Model file for the job. Use its own axes, mm. Face numbers are marked on the shaded views. A direction names the side the tool comes from. Round coordinates to 2 decimals unless told otherwise and drop trailing zeros. Order: outer loops, then holes, each group sorted by start corner. A loop starts at its lowest first (then second) coordinate and runs counter-clockwise, first axis right, second up. Notation, with made-up numbers: (66.25, -6) - (109.25, -6) arc R22 ccw to (109.25, 15) - close; hole circle Ø7 at (19.5, 54.5). An arc over 180 degrees is marked (long way). Put each result on its own line as item: value. Start each with the question number.
Item 1: Saw through at B-B on x = -18. List the corners of the cut face in (y, z).
Item 2: Which spindle directions (+Z, -Z, +X, -X, +Y, -Y) get a long thin tool onto all of the face, cutting with end or side? Do the marked faces 1, 2 and 3. Say none if no direction does.
Item 3: Mould opens along Y. For the marked faces 4, 5 and 6 say: pulls with the +Y half, pulls with the -Y half, needs draft (parallel to the pull), parting line crosses it, or undercut.
Item 4: Pin check, flat tips, straight feed: pin 1 Ø5.5 at (x, z) = (-23.5, 22) entering from -Y; pin 2 Ø0.6 at (y, z) = (6.5, 16.5) entering from +X; pin 3 Ø1.5 at (y, z) = (1.5, 16.5) entering from +X; pin 4 Ø1.4 at (y, z) = (7, 7) entering from +X. Stop position of each tip, or through.
Item 5: Saw through at A-A on y = 0. State how many separate pieces and enclosed holes the cut face has, plus the area to 3 significant figures.
Item 6: Saw through at C-C on z = 21.5. List the corners of the cut face in (x, y), plus the area to 3 significant figures.
Item 7: Saw through at D-D on x = -30. List the corners of the cut face in (y, z), plus the area to 3 significant figures.
Item 8: Probe probe 1 along Y at (x, z) = (0, 0.9); probe 2 along Y at (x, z) = (-23, 19); probe 3 along Z at (x, y) = (-30, 3.5). List the from-to ranges inside material, lowest first.
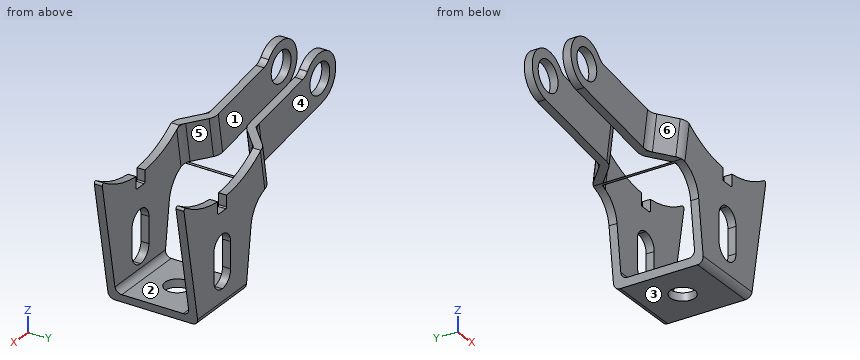
```python
from build123d import *

# Parameters (mm, degrees)
F1_DEPTH       = 7.3
F1_DEPTH_BACK  = 7.3
F3_DEPTH       = 6
F3_DEPTH_BACK  = 6
F5_DEPTH       = 10
F5_DEPTH_BACK  = 10
F8_DEPTH       = 25
F9_R           = 2.5
F10_DEPTH      = 10
F10_DEPTH_BACK = 10
F11_T1_DEPTH   = 6.5
F11_T6_DEPTH   = 12.7132034356
F11_S7_R       = 5
F11_T8_DEPTH   = 8
F11_S10_R      = 17
F11_T11_DEPTH  = 8
F11_T15_DEPTH  = 8.5710678119
F11_T20_DEPTH  = 12.7132034356
F11_S21_R      = 5
F11_T22_DEPTH  = 8
F11_S24_R      = 17
F11_T25_DEPTH  = 8
F11_T29_DEPTH  = 8.5710678119
F11_T31_DEPTH  = 10.6421356237
F12_R          = 1
F13_R          = 2
F14_DEPTH      = 5


# Not quite as in the source:
# - a fillet or chamfer that OpenCascade refuses, or shapes differently, is made with other operations: its cross-section is extruded or revolved along the edge and cut away or added


with BuildPart() as f1:
    # F0 (on Front) → F1 (new body, two sides)
    with BuildSketch(Plane.XZ) as f1_sk:
        with BuildLine():
            Line((-7.2480415045, 9.479816391), (-6, 0))
            Line((-6, 0), (6, 0))
            Line((6, 0), (9.6197658273, 19.3731186918))
            ThreePointArc((9.6197658273, 19.3731186918), (9.492555749, 19.6769779623), (9.1631662961, 19.6809084286))
            ThreePointArc((9.1631662961, 19.6809084286), (-0.3536100614, 17.0036780472), (-9.750799418, 20.0744152471))
            Line((-9.750799418, 20.0744152471), (-25.666835692, 22.7954629152))
            ThreePointArc((-25.666835692, 22.7954629152), (-26.3420622378, 23.0419468668), (-26.8865335991, 23.511240126))
            ThreePointArc((-26.8865335991, 23.511240126), (-33.4498266444, 23.0245236782), (-30.6740705867, 17.0572054525))
            Line((-30.6740705867, 17.0572054525), (-11.362677578, 13.7556786143))
            ThreePointArc((-11.362677578, 13.7556786143), (-8.6024605414, 12.2941429125), (-7.2480415045, 9.479816391))
        make_face()
    extrude(amount=F1_DEPTH)
    extrude(f1_sk.sketch, amount=-F1_DEPTH_BACK)

    # F2 (on Front) → F3 (cut, two sides)
    with BuildSketch(Plane.XZ) as f3_sk:
        Polygon((15, 1.3), (15, 78.0352148958), (0, 78.0352148958), (-11, 13.6936742961), (-11, 1.3), align=None)
    extrude(amount=F3_DEPTH, mode=Mode.SUBTRACT)
    extrude(f3_sk.sketch, amount=-F3_DEPTH_BACK, mode=Mode.SUBTRACT)

    # F4 (on Front) → F5 (cut, two sides)
    with BuildSketch(Plane.XZ) as f5_sk:
        with BuildLine():
            Line((0, 18), (-1.125, 18))
            Line((-1.125, 18), (-1.125, 15.2))
            ThreePointArc((-1.125, 15.2), (-1.0664213562, 15.0585786438), (-0.925, 15))
            Line((-0.925, 15), (0, 15))
            Line((0, 15), (0.925, 15))
            ThreePointArc((0.925, 15), (1.0664213562, 15.0585786438), (1.125, 15.2))
            Line((1.125, 15.2), (1.125, 18))
            Line((1.125, 18), (0, 18))
        make_face()
        with BuildLine():
            ThreePointArc((0, 11.5), (-1.50260191, 10.87760191), (-2.125, 9.375))
            Line((-2.125, 9.375), (-2.125, 5.125))
            ThreePointArc((-2.125, 5.125), (-1.50260191, 3.62239809), (0, 3))
            ThreePointArc((0, 3), (1.50260191, 3.62239809), (2.125, 5.125))
            Line((2.125, 5.125), (2.125, 9.375))
            ThreePointArc((2.125, 9.375), (1.50260191, 10.87760191), (0, 11.5))
        make_face()
    extrude(amount=F5_DEPTH, mode=Mode.SUBTRACT)
    extrude(f5_sk.sketch, amount=-F5_DEPTH_BACK, mode=Mode.SUBTRACT)

    # F7 (on offset) → F8 (cut)
    with BuildSketch(Plane(origin=(1.9622434031, 0, 11.4776148716), x_dir=(0.9856986369, 0, -0.1685176467), z_dir=(-0.1685176467, 0, -0.9856986369))):
        Polygon((-41.9907133171, -7.3), (-13.6887884036, -7.3), (-17.1887884036, -3.8), (-41.9907133171, -3.8), align=None)
        Polygon((-41.9907133171, 7.3), (-41.9907133171, 3.8), (-17.1887884036, 3.8), (-13.6887884036, 7.3), align=None)
        Polygon((-16.6503107725, -2.5), (-13.1503107725, -6), (-13.1503107725, 0), (-13.1503107725, 6), (-16.6503107725, 2.5), (-41.9907133171, 2.5), (-41.9907133171, 0), (-41.9907133171, -2.5), align=None)
    extrude(amount=-F8_DEPTH, mode=Mode.SUBTRACT)

    # F9 (on Front) → F10 (cut, two sides)
    with BuildSketch(Plane.XZ) as f10_sk:
        with Locations((-30, 21)):
            Circle(F9_R)
    extrude(amount=F10_DEPTH, mode=Mode.SUBTRACT)
    extrude(f10_sk.sketch, amount=-F10_DEPTH_BACK, mode=Mode.SUBTRACT)

    # F11: fillet of radius 2 on 8 edges, made by hand

    # F11_s2 → F11_t1 (join)
    with BuildSketch(Plane(origin=(1.9622434031, 0, 11.4776148716), x_dir=(0, 1, 0), z_dir=(0.1685176467, 0, 0.9856986369))):
        with BuildLine():
            ThreePointArc((3.8, 18.0172155284), (3.952240935, 17.2518486636), (4.3857864376, 16.603001966))
            Line((4.3857864376, 16.603001966), (3.8, 17.1887884036))
            Line((3.8, 17.1887884036), (3.8, 18.0172155284))
        make_face()
        with BuildLine():
            ThreePointArc((-4.3857864376, 16.603001966), (-3.952240935, 17.2518486636), (-3.8, 18.0172155284))
            Line((-3.8, 18.0172155284), (-3.8, 17.1887884036))
            Line((-3.8, 17.1887884036), (-4.3857864376, 16.603001966))
        make_face()
    extrude(amount=F11_T1_DEPTH)


with BuildPart() as f11_tool4:
    # F11_s5 → F11_t6 (new body)
    with BuildSketch(Plane(origin=(3.0576081065, 0, 17.8846560114), x_dir=(0, 1, 0), z_dir=(-0.1685176467, 0, -0.9856986369))):
        with BuildLine():
            ThreePointArc((-6, -12.3218836478), (-5.847759065, -13.0872505125), (-5.4142135624, -13.7360972102))
            Line((-5.4142135624, -13.7360972102), (-6, -13.1503107725))
            Line((-6, -13.1503107725), (-6, -12.3218836478))
        make_face()
    extrude(amount=F11_T6_DEPTH)

    # F11_s7 → F11_t8 (cut, symmetric)
    with BuildSketch(Plane.XZ.offset(5.7)):
        with Locations((-12.2052658114, 8.8271854299)):
            Circle(F11_S7_R)
    extrude(amount=F11_T8_DEPTH, both=True, mode=Mode.SUBTRACT)

    split(bisect_by=Plane.YZ.offset(-11), keep=Keep.TOP)

    # F11_s10 → F11_t11 (cut, symmetric)
    with BuildSketch(Plane.XZ.offset(5.7)):
        with Locations((0, 34)):
            Circle(F11_S10_R)
    extrude(amount=F11_T11_DEPTH, both=True, mode=Mode.SUBTRACT)


with BuildPart() as f1_1:
    add(f1.part)

    # F11_t3: union F11_tool4
    add(f11_tool4.part)


with BuildPart() as f11_tool13:
    # F11_s14 → F11_t15 (new body)
    with BuildSketch(Plane(origin=(3.4066195803, 0, 19.9261047304), x_dir=(0, 1, 0), z_dir=(-0.1685176467, 0, -0.9856986369))):
        with BuildLine():
            ThreePointArc((-6, -12.3218836478), (-5.847759065, -13.0872505125), (-5.4142135624, -13.7360972102))
            Line((-5.4142135624, -13.7360972102), (-6, -13.1503107725))
            Line((-6, -13.1503107725), (-6, -12.3218836478))
        make_face()
    extrude(amount=F11_T15_DEPTH)

    split(bisect_by=Plane.YZ.offset(-11), keep=Keep.BOTTOM)


with BuildPart() as f1_2:
    add(f1_1.part)

    # F11_t12: union F11_tool13
    add(f11_tool13.part)


with BuildPart() as f11_tool18:
    # F11_s19 → F11_t20 (new body)
    with BuildSketch(Plane(origin=(3.0576081065, 0, 17.8846560114), x_dir=(0, 1, 0), z_dir=(-0.1685176467, 0, -0.9856986369))):
        with BuildLine():
            ThreePointArc((6, -12.3218836478), (5.847759065, -13.0872505125), (5.4142135624, -13.7360972102))
            Line((5.4142135624, -13.7360972102), (6, -13.1503107725))
            Line((6, -13.1503107725), (6, -12.3218836478))
        make_face()
    extrude(amount=F11_T20_DEPTH)

    # F11_s21 → F11_t22 (cut, symmetric)
    with BuildSketch(Plane.XZ.offset(-5.7)):
        with Locations((-12.2052658114, 8.8271854299)):
            Circle(F11_S21_R)
    extrude(amount=F11_T22_DEPTH, both=True, mode=Mode.SUBTRACT)

    split(bisect_by=Plane.YZ.offset(-11), keep=Keep.TOP)

    # F11_s24 → F11_t25 (cut, symmetric)
    with BuildSketch(Plane.XZ.offset(-5.7)):
        with Locations((0, 34)):
            Circle(F11_S24_R)
    extrude(amount=F11_T25_DEPTH, both=True, mode=Mode.SUBTRACT)


with BuildPart() as f1_3:
    add(f1_2.part)

    # F11_t17: union F11_tool18
    add(f11_tool18.part)


with BuildPart() as f11_tool27:
    # F11_s28 → F11_t29 (new body)
    with BuildSketch(Plane(origin=(3.4066195803, 0, 19.9261047304), x_dir=(0, 1, 0), z_dir=(-0.1685176467, 0, -0.9856986369))):
        with BuildLine():
            ThreePointArc((6, -12.3218836478), (5.847759065, -13.0872505125), (5.4142135624, -13.7360972102))
            Line((5.4142135624, -13.7360972102), (6, -13.1503107725))
            Line((6, -13.1503107725), (6, -12.3218836478))
        make_face()
    extrude(amount=F11_T29_DEPTH)

    split(bisect_by=Plane.YZ.offset(-11), keep=Keep.BOTTOM)


with BuildPart() as f1_4:
    add(f1_3.part)

    # F11_t26: union F11_tool27
    add(f11_tool27.part)

    # F11_s32 → F11_t31 (cut)
    with BuildSketch(Plane(origin=(1.6132319293, 0, 9.4361661525), x_dir=(0, 1, 0), z_dir=(0.1685176467, 0, 0.9856986369))):
        with BuildLine():
            ThreePointArc((6.7142135624, 14.2745748413), (7.147759065, 13.6257281436), (7.3, 12.8603612789))
            Line((7.3, 12.8603612789), (7.3, 13.6887884036))
            Line((7.3, 13.6887884036), (6.7142135624, 14.2745748413))
        make_face()
        with BuildLine():
            ThreePointArc((-2.5, 17.4787378973), (-2.652240935, 16.7133710326), (-3.0857864376, 16.0645243349))
            Line((-3.0857864376, 16.0645243349), (-2.5, 16.6503107725))
            Line((-2.5, 16.6503107725), (-2.5, 17.4787378973))
        make_face()
        with BuildLine():
            ThreePointArc((-6.7142135624, 14.2745748413), (-7.147759065, 13.6257281436), (-7.3, 12.8603612789))
            Line((-7.3, 12.8603612789), (-7.3, 13.6887884036))
            Line((-7.3, 13.6887884036), (-6.7142135624, 14.2745748413))
        make_face()
        with BuildLine():
            ThreePointArc((2.5, 17.4787378973), (2.652240935, 16.7133710326), (3.0857864376, 16.0645243349))
            Line((3.0857864376, 16.0645243349), (2.5, 16.6503107725))
            Line((2.5, 16.6503107725), (2.5, 17.4787378973))
        make_face()
    extrude(amount=F11_T31_DEPTH, mode=Mode.SUBTRACT)

    # F12
    f12_edges = [f1_4.edges().sort_by_distance(p)[0] for p in [
        (0.035875, 6, 1.3),
        (0, -7.3, 0),
        (0.035875, -6, 1.3),
        (0, 7.3, 0),
    ]]
    fillet(f12_edges, radius=F12_R)

    # F13 (on Top) → F14 (cut)
    with BuildSketch(Plane.XY):
        Circle(F13_R)
    extrude(amount=F14_DEPTH, mode=Mode.SUBTRACT)


solid = f1_4.part
```
Results found:
1. outline: (-3.8, 14.89) - (-2.5, 14.89) - (-2.5, 21.48) - (-3.8, 21.48) - close; (2.5, 14.89) - (3.8, 14.89) - (3.8, 21.48) - (2.5, 21.48) - close
2. face 1: +Z, -Z, +X, -X
2. face 2: +Z, +X, -X
2. face 3: -Z, +X, -X, +Y, -Y
3. face 4: pulls with the +Y half
3. face 5: undercut
3. face 6: pulls with the -Y half
4. pin 1: stops at y = -3.8
4. pin 2: stops at x = 9.14
4. pin 3: passes through
4. pin 4: stops at x = 7.44
5. separate pieces: 3
5. enclosed holes: 0
5. area: 10.7 mm²
6. outline: (-33.97, -3.8) - (-32.45, -3.8) - (-32.45, -2.5) - (-33.97, -2.5) - close; (-33.97, 2.5) - (-32.45, 2.5) - (-32.45, 3.8) - (-33.97, 3.8) - close; (-27.55, -3.8) - (-18.09, -3.8) - (-18.09, -2.5) - (-27.55, -2.5) - close; (-27.55, 2.5) - (-18.09, 2.5) - (-18.09, 3.8) - (-27.55, 3.8) - close
6. area: 28.5 mm²
7. outline: (-3.8, 16.94) - (-2.5, 16.94) - (-2.5, 18.5) - (-3.8, 18.5) - close; (-3.8, 23.5) - (-2.5, 23.5) - (-2.5, 25) - (-3.8, 25) - close; (2.5, 16.94) - (3.8, 16.94) - (3.8, 18.5) - (2.5, 18.5) - close; (2.5, 23.5) - (3.8, 23.5) - (3.8, 25) - (2.5, 25) - close
7. area: 7.95 mm²
8. probe 1: y = -7.29 to -2, 2 to 7.29
8. probe 2: y = -3.8 to -2.5, 2.5 to 3.8
8. probe 3: z = 16.94 to 18.5, 23.5 to 25
